Read the model definition and answer for the solid it produces. Units are mm, in the model's axes. Face numbers are marked on the shaded views. Coordinates: 2 decimals unless noted, no trailing zeros. Loops run counter-clockwise (first coordinate to the right, second up) from the corner with the lowest first, then second, coordinate; pieces in that order, holes last. Notation, with made-up numbers: (60, -39) -> (111, -39) arc R8 ccw to (111, -32) -> close; hole circle Ø10 at (-37, 85.25). An arc over 180 degrees is marked (long way). Answer as CSV lines item,"result".
```python
from build123d import *

# Parameters (mm, degrees)
SZKIC1_R                        = 12
SZKIC1_R_2                      = 6
DODANIE_WYCI_GNI_CIE1_DEPTH     = 40
SZKIC2_R                        = 12
DODANIE_WYCI_GNI_CIE2_DEPTH     = 23
SZKIC3_R                        = 20
DODANIE_WYCI_GNI_CIE3_DEPTH     = 200
SZKIC4_R                        = 15
WYTNIJ_WYCI_GNI_CIE1_DEPTH      = 150
WYTNIJ_WYCI_GNI_CIE2_DEPTH      = 250
WYTNIJ_WYCI_GNI_CIE2_DEPTH_BACK = 250
SZKIC5_R                        = 5


with BuildPart() as part:
    # Szkic1 → Dodanie-wyci_gni_cie1 (new body)
    with BuildSketch(Plane.XY):
        Circle(SZKIC1_R)
        Circle(SZKIC1_R_2, mode=Mode.SUBTRACT)
    extrude(amount=DODANIE_WYCI_GNI_CIE1_DEPTH)

    # Szkic2 → Dodanie-wyci_gni_cie2 (add)
    with BuildSketch(Plane.XY.offset(40)):
        Circle(SZKIC2_R)
    extrude(amount=DODANIE_WYCI_GNI_CIE2_DEPTH)

    # Szkic3 → Dodanie-wyci_gni_cie3 (add)
    with BuildSketch(Plane.XY.offset(63)):
        Circle(SZKIC3_R)
    extrude(amount=DODANIE_WYCI_GNI_CIE3_DEPTH)

    # Szkic4 → Wytnij-wyci_gni_cie1 (cut)
    with BuildSketch(Plane.XY.offset(263)):
        Circle(SZKIC4_R)
    extrude(amount=-WYTNIJ_WYCI_GNI_CIE1_DEPTH, mode=Mode.SUBTRACT)

    # Szkic5 → Wytnij-wyci_gni_cie2 (cut, two sides: drawn at the far end of the back side and taken through both)
    with BuildSketch(Plane(origin=(0, 0, 0), x_dir=(1, 0, 0), z_dir=(0, 1, 0)).offset(-WYTNIJ_WYCI_GNI_CIE2_DEPTH_BACK)):
        with Locations((0, -333.024962479)):
            Circle(SZKIC5_R)
        with Locations((0, -293.024962479)):
            Circle(SZKIC5_R)
        with Locations(Location((0, -253.024962479, 0), (0, 0, 90))):
            Circle(SZKIC5_R)
        with Locations(Location((0, -213.024962479, 0), (0, 0, 90))):
            Circle(SZKIC5_R)
        with Locations(Location((0, -173.024962479, 0), (0, 0, 90))):
            Circle(SZKIC5_R)
    extrude(amount=WYTNIJ_WYCI_GNI_CIE2_DEPTH + WYTNIJ_WYCI_GNI_CIE2_DEPTH_BACK, mode=Mode.SUBTRACT)


solid = part.part
```
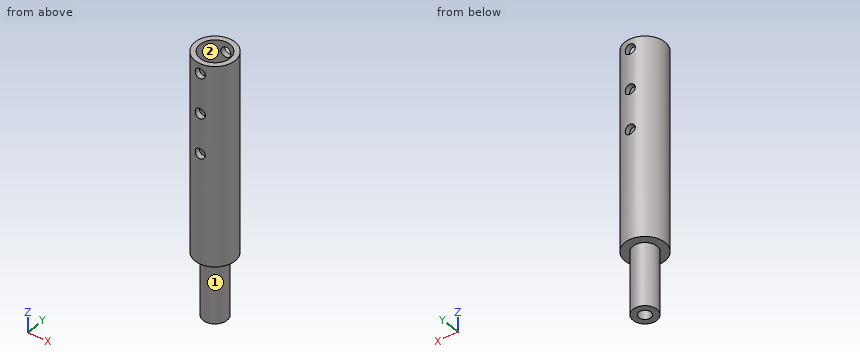
Q1. A cutting plane is placed at A-A, the plane y = 0. Write down the section's boundary in (x, z), and give its area (3 significant figures).
Results:
outline,"(-20, 63) -> (-12, 63) -> (-12, 0) -> (-6, 0) -> (-6, 40) -> (6, 40) -> (6, 0) -> (12, 0) -> (12, 63) -> (20, 63) -> (20, 263) -> (15, 263) -> (15, 113) -> (-15, 113) -> (-15, 263) -> (-20, 263) -> close"
area,"4,530 mm²"
Q2. For a pull along X with two mould halves and no side action, classify the marked faces 1 and 2 as pulls with the +X half, pulls with the -X half, needs draft (parallel to the pull), parting line crosses it, or undercut.
Results:
face 1,"parting line crosses it"
face 2,"undercut"
Q3. Find the intervals of material crossed by probe 1 along Z at (x, y) = (17, 8); probe 2 along X at (y, z) = (7, 121.5) (1 decimal); probe 3 along Y at (x, z) = (-9, 207.5), in increasing order. Write a range as [from, to].
Results:
probe 1,"z = [63, 263]"
probe 2,"x = [-18.7, -13.3], [13.3, 18.7]"
probe 3,"y = [-17.86, -12], [12, 17.86]"
Q4. A cutting plane is placed at B-B, the plane z = 132. Write down the section's boundary in (x, y), and give its area (3 significant figures).
Results:
outline,"circle Ø40 at (0, 0); hole circle Ø30 at (0, 0)"
area,"550 mm²"
Q5. Given pin 1 Ø16 at (x, z) = (0, 173.02) entering from +Y; pin 2 Ø10 at (x, z) = (8.5, 233.5) entering from +Y; pin 3 Ø8 at (x, z) = (0, 213.02) entering from +Y; pin 4 Ø8 at (x, z) = (11, 99.5) entering from +Y (3 decimals), each flat-ended and moving along its own axis, determine where each tip first touches the part or whether it passes through.
Results:
pin 1,"stops at y = 20"
pin 2,"stops at y = 19.69"
pin 3,"passes through"
pin 4,"stops at y = 18.735"
Q6. A cutting plane is placed at C-C, the plane x = 0. Give the number of separate pieces and of enclosed holes in the cut face, and give its area (3 significant figures).
Results:
separate pieces,"7"
enclosed holes,"0"
area,"4,230 mm²"
